Geometry: final body of the model. Coordinates: model frame, mm. Face numbers are marked on the shaded views. Coordinates: 2 decimals unless noted, no trailing zeros. Use a Markdown table: item, result. Add a question column.
```python
from build123d import *

# Parameters (mm, degrees)
F0_W     = 54.224986
F0_H     = 23.8125
F0_R     = 6.000001
F1_DEPTH = 12.349988
F2_R     = 7.999997
F3_DEPTH = 3.175
F4_R     = 7.999997
F5_DEPTH = 3.175
F6_R     = 2.15265
F7_DEPTH = 23.8125
F8_SIZE  = 0.508


with BuildPart() as f1:
    # F0 (on Top) → F1 (new body)
    with BuildSketch(Plane.XY):
        Rectangle(F0_W, F0_H)
        with Locations((-9.587497, 0)):
            Circle(F0_R, mode=Mode.SUBTRACT)
        with Locations((9.587497, 0)):
            Circle(F0_R, mode=Mode.SUBTRACT)
    extrude(amount=F1_DEPTH)

    # F2 (on face) → F3 (cut)
    with BuildSketch(Plane(origin=(0, 0, 0), x_dir=(1, 0, 0), z_dir=(0, 0, -1))):
        with Locations((9.587497, 0)):
            Circle(F2_R)
        with Locations((-9.587497, 0)):
            Circle(F2_R)
    extrude(amount=-F3_DEPTH, mode=Mode.SUBTRACT)

    # F4 (on face) → F5 (cut)
    with BuildSketch(Plane.XY.offset(12.349988)):
        with Locations((9.587497, 0)):
            Circle(F4_R)
        with Locations((-9.587497, 0)):
            Circle(F4_R)
    extrude(amount=-F5_DEPTH, mode=Mode.SUBTRACT)

    # F6 (on face) → F7 (cut, through all)
    with BuildSketch(Plane.XZ.offset(11.90625)):
        with Locations((-22.349993, 6.174994)):
            Circle(F6_R)
        with Locations((22.349993, 6.174994)):
            Circle(F6_R)
    extrude(amount=-F7_DEPTH, mode=Mode.SUBTRACT)

    # F8
    f8_edges = [f1.edges().sort_by_distance(p)[0] for p in [
        (1.5875, 0, 0),
        (3.587496, 0, 3.175),
        (3.587496, 0, 9.174988),
        (1.5875, 0, 12.349988),
        (-17.587493, 0, 12.349988),
        (-17.587493, 0, 0),
        (-15.587497, 0, 3.175),
        (-15.587497, 0, 9.174988),
    ]]
    chamfer(f8_edges, length=F8_SIZE)


solid = f1.part
```
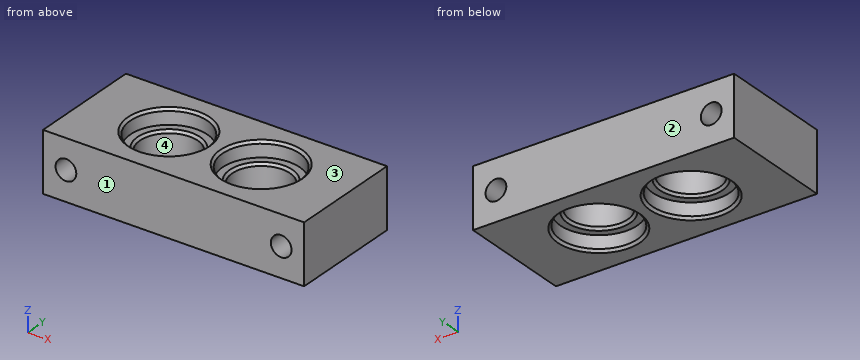
1) First-contact query: pin 1 (7 mm diameter, centred on x = -9.59, y = 0, fed in from +Z); pin 2 (14 mm diameter, centred on x = 9.59, y = 0, fed in from -Z) (3 decimals). Flat tips, straight axial feed; report the tip coordinate or a pass-through.
2) Line query: line 1 (X direction, y = 0, z = 1.9); line 2 (X direction, y = 10.25, z = 5); line 3 (X direction, y = -4, z = 7.25) (1 decimal). Output: solid intervals per line, ascending. Write a range as from..to.
3) Draft query along Y for the marked faces 1, 2, 3 and 4. Return one class per face: released by +Y, released by -Y, zero draft, split by the parting line, or undercut.
4) Section query A-A (y = -2.5). Give the number of separate pieces and of enclosed holes in the cut face, and give its area (3 significant figures).
From the geometry:
| question | item | result |
|---|---|---|
| 1 | pin 1 | passes through |
| 1 | pin 2 | stops at z = 3.175 |
| 2 | line 1 | x = -27.11..-17.59, -1.59..1.59, 17.59..27.11 |
| 2 | line 2 | x = -27.11..-24.15, -20.55..20.55, 24.15..27.11 |
| 2 | line 3 | x = -27.1..-24.2, -20.5..-14.1, -5.1..5.1, 14.1..20.5, 24.2..27.1 |
| 3 | face 1 | released by -Y |
| 3 | face 2 | released by +Y |
| 3 | face 3 | zero draft |
| 3 | face 4 | undercut |
| 4 | separate pieces | 3 |
| 4 | enclosed holes | 2 |
| 4 | area | 314 mm^2 |
